Here's how the part is built. I have some questions about the finished solid (model axes, mm). A direction names the side the tool comes from. Give positions to 0.01 mm unless a question says otherwise; leave off trailing zeros. Order: outer loops, then holes, each group sorted by start corner. A loop starts at its lowest first (then second) coordinate and runs counter-clockwise, first axis right, second up. Notation, with made-up numbers: M 88.25,-18 L 103.25,-18 A16 cw 103.25,2 Z; hole C -14.75,62.25 d5. An arc over 180 degrees is marked long. Use one line per item in the form item = value.
from build123d import *

# Parameters (mm, degrees)
F1_DEPTH = 3.175
F3_DEPTH = 50


with BuildPart() as f1:
    # F0 (on Top) → F1 (new body)
    with BuildSketch(Plane.XY):
        with BuildLine():
            Line((0, 3.37345), (0, 6))
            ThreePointArc((0, 6), (-4.2426406871, 4.2426406871), (-6, 0))
            Line((-6, 0), (-3.37345, 0))
            ThreePointArc((-3.37345, 0), (-2.385389371, 2.385389371), (0, 3.37345))
        make_face()
        with BuildLine():
            Line((0, 0), (0, 3.37345))
            ThreePointArc((0, 3.37345), (-2.385389371, 2.385389371), (-3.37345, 0))
            Line((-3.37345, 0), (0, 0))
        make_face()
        with BuildLine():
            ThreePointArc((3.37345, 0), (2.385389371, 2.385389371), (0, 3.37345))
            Line((0, 3.37345), (0, 0))
            Line((0, 0), (3.37345, 0))
        make_face()
        with BuildLine():
            ThreePointArc((6, 0), (4.2426406871, 4.2426406871), (0, 6))
            Line((0, 6), (0, 3.37345))
            ThreePointArc((0, 3.37345), (2.385389371, 2.385389371), (3.37345, 0))
            Line((3.37345, 0), (6, 0))
        make_face()
        with BuildLine():
            ThreePointArc((0, -6), (4.2426406871, -4.2426406871), (6, 0))
            Line((6, 0), (3.37345, 0))
            ThreePointArc((3.37345, 0), (2.385389371, -2.385389371), (0, -3.37345))
            Line((0, -3.37345), (0, -6))
        make_face()
        with BuildLine():
            Line((3.37345, 0), (0, 0))
            Line((0, 0), (0, -3.37345))
            ThreePointArc((0, -3.37345), (2.385389371, -2.385389371), (3.37345, 0))
        make_face()
        with BuildLine():
            Line((0, -3.37345), (0, 0))
            Line((0, 0), (-3.37345, 0))
            ThreePointArc((-3.37345, 0), (-2.385389371, -2.385389371), (0, -3.37345))
        make_face()
        with BuildLine():
            Line((-3.37345, 0), (-6, 0))
            ThreePointArc((-6, 0), (-4.2426406871, -4.2426406871), (0, -6))
            Line((0, -6), (0, -3.37345))
            ThreePointArc((0, -3.37345), (-2.385389371, -2.385389371), (-3.37345, 0))
        make_face()
    extrude(amount=-F1_DEPTH)

    # F2 (on Top) → F3 (join)
    with BuildSketch(Plane.XY):
        with BuildLine():
            ThreePointArc((3.37345, 0), (2.385389371, 2.385389371), (0, 3.37345))
            Line((0, 3.37345), (0, 0))
            Line((0, 0), (3.37345, 0))
        make_face()
        with BuildLine():
            Line((3.37345, 0), (0, 0))
            Line((0, 0), (0, -3.37345))
            ThreePointArc((0, -3.37345), (2.385389371, -2.385389371), (3.37345, 0))
        make_face()
        with BuildLine():
            Line((0, -3.37345), (0, 0))
            Line((0, 0), (-3.37345, 0))
            ThreePointArc((-3.37345, 0), (-2.385389371, -2.385389371), (0, -3.37345))
        make_face()
        with BuildLine():
            Line((0, 0), (0, 3.37345))
            ThreePointArc((0, 3.37345), (-2.385389371, 2.385389371), (-3.37345, 0))
            Line((-3.37345, 0), (0, 0))
        make_face()
    extrude(amount=F3_DEPTH)


solid = f1.part
Q1. On a 3-axis mill with a long thin cutter (end or side, diameter ignored), from which of +Z, -Z, +X, -X, +Y, -Y can I reach the whole of each face in a straight line? I mean faces 1 (the face through (0, 0, -3.175)), 2 (the face through (3, -3, 0)). Say none if no direction works.
Found:
face_1 = -Z, +X, -X, +Y, -Y
face_2 = +Z
Q2. I need wall thicknesses on L1, parallel to Z at x = 2, y = -3.5 (3 decimals); L2, parallel to Y at x = -0.25, z = 27; L3, parallel to X at y = -0.5, z = 5. Which ranges of each line are inside material? Lowest first, please.
Found:
L1 = -3.175 to 0
L2 = -3.36 to 3.36
L3 = -3.34 to 3.34
Q3. I want a section at D-D on y = -5. Write out the boundary of the cut face in (x, z) (3 decimals).
Found:
outline = M -3.317,-3.175 L 3.317,-3.175 L 3.317,0 L -3.317,0 Z
Q4. I want a section at B-B on x = -2.5. Write out the boundary of the cut face in (y, z) (3 decimals).
Found:
outline = M -5.454,-3.175 L 5.454,-3.175 L 5.454,0 L 2.265,0 L 2.265,50 L -2.265,50 L -2.265,0 L -5.454,0 Z
Q5. I want a section at C-C on z = 20.5. Write out the boundary of the cut face in (x, y).
Found:
outline = C 0,0 d6.75
Q6. I'm going to push flat-ended pins straight in: pin 1 Ø5 at (x, z) = (-2.5, 8) entering from +Y; pin 2 Ø1.5 at (x, y) = (0, -4) entering from +Z; pin 3 Ø4 at (y, z) = (3.5, 5) entering from -X; pin 4 Ø5 at (y, z) = (-3, 34) entering from +X. Where does each tip first touch, or does it pass through?
Found:
pin_1 = 3.37
pin_2 = 50
pin_3 = -3.02
pin_4 = 3.34
Q7. I want a section at A-A on y = -2.75. Write out the boundary of the cut face in (x, z) (3 decimals), then the cut area to 3 significant figures.
Found:
outline = M -5.333,-3.175 L 5.333,-3.175 L 5.333,0 L 1.954,0 L 1.954,50 L -1.954,50 L -1.954,0 L -5.333,0 Z
area = 229 mm²
